```python
from build123d import *

# Parameters (mm, degrees)
BOSS_EXTRUDE1_DEPTH     = 20
SKETCH4_R               = 2.55
CUT_EXTRUDE2_DEPTH      = 34.212108316
CUT_EXTRUDE3_DEPTH      = 34.212108316
CUT_EXTRUDE3_DEPTH_BACK = 34.212108316
SKETCH5_R               = 2.55
SKETCH6_R               = 5.3
CUT_EXTRUDE4_DEPTH      = 17
CUT_EXTRUDE5_DEPTH      = 7
CUT_EXTRUDE5_DEPTH_BACK = 10
SKETCH7_R               = 5.3
FILLET1_R               = 0.7
FILLET2_R               = 3


with BuildPart() as part:
    # Sketch1 → Boss-Extrude1 (new body)
    with BuildSketch(Plane.XY):
        Polygon((-10, 13.094), (9.854423989, 24.556957035), (9.854423989, 1.462957035), (-10, -10), align=None)
    extrude(amount=BOSS_EXTRUDE1_DEPTH)

    # Sketch4 → Cut-Extrude2 (cut, through all)
    with BuildSketch(Plane.XY):
        with Locations((-0.072788005, 7.278478517)):
            Circle(SKETCH4_R)
    extrude(amount=CUT_EXTRUDE2_DEPTH, mode=Mode.SUBTRACT)

    # Sketch5 → Cut-Extrude3 (cut, two sides: drawn at the far end of the back side and taken through both)
    with BuildSketch(Plane(origin=(0, 0, 0), x_dir=(0, 0, -1), z_dir=(1, 0, 0)).offset(-CUT_EXTRUDE3_DEPTH_BACK)):
        with Locations((-10, 7.278478517)):
            Circle(SKETCH5_R)
    extrude(amount=CUT_EXTRUDE3_DEPTH + CUT_EXTRUDE3_DEPTH_BACK, mode=Mode.SUBTRACT)

    # Sketch6 → Cut-Extrude4 (cut)
    with BuildSketch(Plane.XY):
        with Locations((-0.072788005, 7.278478517)):
            Circle(SKETCH6_R)
    extrude(amount=CUT_EXTRUDE4_DEPTH, mode=Mode.SUBTRACT)

    # Sketch7 → Cut-Extrude5 (cut, two sides: drawn at the far end of the back side and taken through both)
    with BuildSketch(Plane(origin=(0, 0, 0), x_dir=(0, 0, -1), z_dir=(1, 0, 0)).offset(-CUT_EXTRUDE5_DEPTH_BACK)):
        with Locations(Location((-10, 7.278478517, 0), (0, 0, 90))):
            Circle(SKETCH7_R)
    extrude(amount=CUT_EXTRUDE5_DEPTH + CUT_EXTRUDE5_DEPTH_BACK, mode=Mode.SUBTRACT)

    # Fillet1
    fillet1_edges = [part.edges().sort_by_distance(p)[0] for p in [
        (-5.372788005, 7.278478517, 17),
        (7, 1.978478517, 10),
    ]]
    fillet(fillet1_edges, radius=FILLET1_R)

    # Fillet2
    # the kernel refuses this fillet: 3 mm, written as the material it takes off along each edge
    with BuildSketch(Plane(origin=(-7, -4.803847577, 3), x_dir=(-1, 0, 0), z_dir=(0, 0, -1))) as fillet2_piece_1_section:
        Polygon((0, 0), (FILLET2_R, 0), (FILLET2_R, -FILLET2_R * 1.73205080757), (-FILLET2_R * 0.5, -FILLET2_R * 0.866025403784), align=None)
    fillet2_piece_1 = extrude(amount=FILLET2_R, mode=Mode.PRIVATE)
    fillet2_piece_1 = fillet2_piece_1 - Plane(origin=(-7, -4.803847577, 3), x_dir=(0.49999999999999906, 0.8660254037844392, 0), z_dir=(0, 0, -1)) * Sphere(FILLET2_R, mode=Mode.PRIVATE)
    add(fillet2_piece_1, mode=Mode.SUBTRACT)
    with BuildSketch(Plane(origin=(-7, 11.361949192, 3), x_dir=(-0.5000000000000018, 0.8660254037844377, 0), z_dir=(0, 0, -1))) as fillet2_piece_2_section:
        Polygon((0, 0), (FILLET2_R, 0), (FILLET2_R, -FILLET2_R * 0.57735026919), (FILLET2_R * 0.5, -FILLET2_R * 0.866025403784), align=None)
    fillet2_piece_2 = extrude(amount=FILLET2_R, mode=Mode.PRIVATE)
    fillet2_piece_2 = fillet2_piece_2 - Plane(origin=(-7, 11.361949192, 3), x_dir=(0.8660254037844393, -0.49999999999999883, 0), z_dir=(0, 0, -1)) * Sphere(FILLET2_R, mode=Mode.PRIVATE)
    add(fillet2_piece_2, mode=Mode.SUBTRACT)
    with BuildSketch(Plane(origin=(-10, -4.803847577, 0), x_dir=(0, 0, 1), z_dir=(0, 1, 0))) as fillet2_piece_3:
        with BuildLine():
            CenterArc((FILLET2_R, FILLET2_R), FILLET2_R, 180, 90)
            Line((0, FILLET2_R), (0, 0))
            Line((0, 0), (FILLET2_R, 0))
        make_face()
    extrude(amount=16.16579677, mode=Mode.SUBTRACT)
    with BuildSketch(Plane(origin=(-8.5, 13.960025404, 0), x_dir=(0, 0, 1), z_dir=(0.8660254037844377, 0.5000000000000018, 0))) as fillet2_piece_4:
        with BuildLine():
            CenterArc((FILLET2_R, FILLET2_R), FILLET2_R, 180, 90)
            Line((0, FILLET2_R), (0, 0))
            Line((0, 0), (FILLET2_R, 0))
        make_face()
    extrude(amount=28.693863262, mode=Mode.SUBTRACT)
    with BuildSketch(Plane(origin=(16.349614518, 5.212957035, 0), x_dir=(0, 0, 1), z_dir=(-0.866025403784438, -0.5000000000000012, 0))) as fillet2_piece_5:
        with BuildLine():
            CenterArc((FILLET2_R, FILLET2_R), FILLET2_R, 180, 90)
            Line((0, FILLET2_R), (0, 0))
            Line((0, 0), (FILLET2_R, 0))
        make_face()
    extrude(amount=25.229761647, mode=Mode.SUBTRACT)
    with BuildSketch(Plane(origin=(-10, -10, 3), x_dir=(0, 1, 0), z_dir=(0, 0, 1))) as fillet2_piece_6:
        with BuildLine():
            CenterArc((FILLET2_R * 1.73205080757, -FILLET2_R), FILLET2_R, 90, 120)
            Line((FILLET2_R * 0.866025403784, -FILLET2_R * 1.5), (0, 0))
            Line((0, 0), (FILLET2_R * 1.73205080757, 0))
        make_face()
    extrude(amount=29.990381057, mode=Mode.SUBTRACT)
    with BuildSketch(Plane(origin=(-10, 13.094, 3), x_dir=(0.8660254037844375, 0.5000000000000019, 0), z_dir=(0, 0, 1))) as fillet2_piece_7:
        with BuildLine():
            CenterArc((FILLET2_R * 0.57735026919, -FILLET2_R), FILLET2_R, 90, 60)
            Line((-FILLET2_R * 0.288675134595, -FILLET2_R * 0.5), (0, 0))
            Line((0, 0), (FILLET2_R * 0.57735026919, 0))
        make_face()
    extrude(amount=21.330127019, mode=Mode.SUBTRACT)


solid = part.part
```
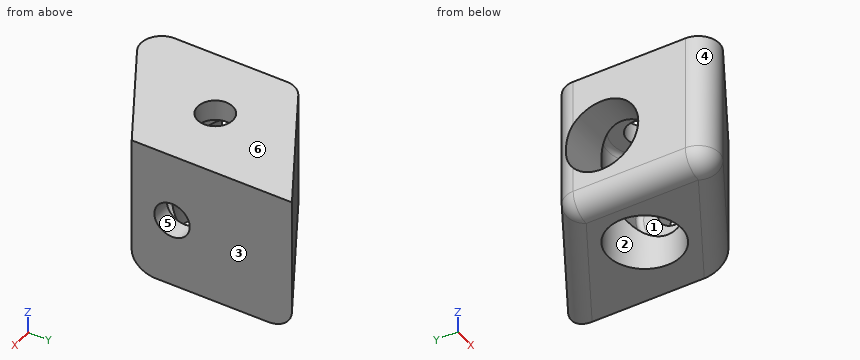
CAD build for the part. Positions are in the model's coordinates, mm. Face numbers are marked on the shaded views. A direction names the side the tool comes from. Round coordinates to 2 decimals unless told otherwise and drop trailing zeros. One line per question, with ' | ' between items.
Q1. Which spindle directions (+Z, -Z, +X, -X, +Y, -Y) get a long thin tool onto all of the face, cutting with end or side? Do the marked faces 1, 2 and 3. Say none if no direction does.
Completed:
face 1: -X | face 2: -Z | face 3: +Z, -Z, +X, +Y, -Y
Q2. Drop flat-ended pins along their axis: pin 1 (4 mm diameter, centred on x = -0.07, y = 7.28, fed in from +Z); pin 2 (6 mm diameter, centred on x = 5, z = 2.5, fed in from -Y); pin 3 (6.5 mm diameter, centred on y = 7.28, z = 10, fed in from -X); pin 4 (5 mm diameter, centred on y = -4.5, z = 13.5, fed in from +X). Give the stop position or say it passes through.
Completed:
pin 1: passes through | pin 2: stops at y = -3.06 | pin 3: stops at x = 7 | pin 4: stops at x = 3.86
Q3. Probe probe 1 along Y at (x, z) = (-5, 10); probe 2 along X at (y, z) = (11, 2.25); probe 3 along Y at (x, z) = (7.75, 12.25). List the from-to ranges inside material, lowest first.
Completed:
probe 1: y = -7.11 to 1.98, 12.58 to 15.98 | probe 2: x = -9.9 to -3.85, 3.7 to 9.85 | probe 3: y = 0.25 to 6.08, 8.48 to 23.34
Q4. Two-plate mould, pull along Y, no slides. Class the marked faces 4, 5 and 6: released by +Y, released by -Y, zero draft, split by the parting line, or undercut.
Completed:
face 4: released by -Y | face 5: undercut | face 6: zero draft
